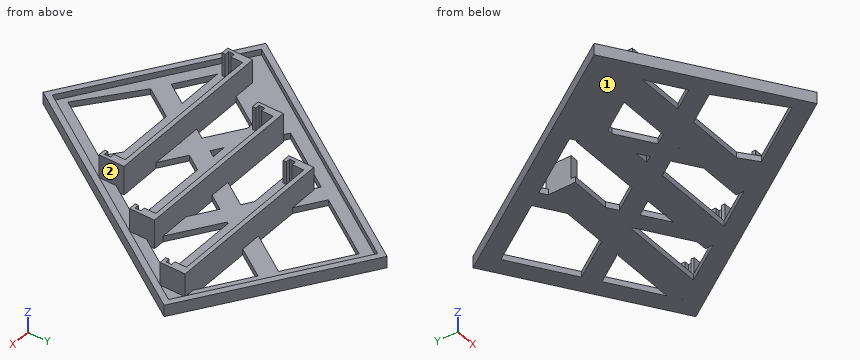
from build123d import *

# Parameters (mm, degrees)
PAD002_DEPTH = 4
PAD001_DEPTH = 10
SKETCH_W     = 59
SKETCH_H     = 10
PAD_DEPTH    = 2
PAD003_DEPTH = 2


with BuildPart() as pad002:
    # Sketch002 → Pad002 (new body)
    with BuildSketch(Plane.XY):
        Polygon((13.415017, 35.19739), (67.498286, -0.858122), (12.028266, -84.063152), (-42.055003, -48.007639), align=None)
        Polygon((13.969717, 32.423889), (-39.281502, -47.452939), (11.473566, -81.289651), (64.724785, -1.412822), align=None, mode=Mode.SUBTRACT)
    extrude(amount=PAD002_DEPTH)


with BuildPart() as pad001:
    # Sketch001 → Pad001 (new body)
    with BuildSketch(Plane.XY):
        Polygon((0, 0), (0, -8.6), (2.6, -8.6), (2.6, -7.5), (1.1, -7.5), (1.1, -5.5), (2.6, -5.5), (2.6, -1.5), (56.4, -1.5), (56.4, -5.5), (57.9, -5.5), (57.9, -7.5), (56.4, -7.5), (56.4, -8.6), (59, -8.6), (59, 0), align=None)
    extrude(amount=PAD001_DEPTH)


with BuildPart() as pad:
    # Sketch → Pad (new body)
    with BuildSketch(Plane.XY):
        with Locations((29.5, -5)):
            Rectangle(SKETCH_W, SKETCH_H)
    extrude(amount=PAD_DEPTH)


with BuildPart() as relay002:
    # Fusion001 base: copy of Pad
    add(pad.part)

    # Fusion001: union Pad001
    add(pad001.part)


with BuildPart() as relay002_1:
    # Fusion001 placement: moved
    add(relay002.part.moved(Location((-14, -21, 0))))


with BuildPart() as relay001:
    # Fusion base: copy of Pad
    add(pad.part)

    # Fusion: union Pad001
    add(pad001.part)


with BuildPart() as relay003:
    # Fusion002 base: copy of Pad
    add(pad.part)

    # Fusion002: union Pad001
    add(pad001.part)


with BuildPart() as relay003_1:
    # Fusion002 placement: moved
    add(relay003.part.moved(Location((-28, -42, 0))))


with BuildPart() as fusion003:
    # Sketch003 → Pad003 (new body)
    with BuildSketch(Plane.XY):
        Polygon((13.415017, 35.19739), (-42.055003, -48.007639), (12.028266, -84.063152), (67.498286, -0.858122), align=None)
        Polygon((15.079117, 26.876888), (34.632299, 13.841433), (20.579895, -7.237174), (1.026713, 5.79828), align=None, mode=Mode.SUBTRACT)
        Polygon((39.624601, 10.513232), (59.177783, -2.522223), (45.125378, -23.60083), (25.572196, -10.565375), align=None, mode=Mode.SUBTRACT)
        Polygon((-2.301489, 0.805979), (-16.353893, -20.272629), (3.199289, -33.308083), (17.251693, -12.229476), align=None, mode=Mode.SUBTRACT)
        Polygon((22.243995, -15.557677), (8.19159, -36.636284), (27.744772, -49.671739), (41.797177, -28.593132), align=None, mode=Mode.SUBTRACT)
        Polygon((0.059977, -38.426311), (-13.992428, -59.504919), (-26.473182, -51.184416), (-12.420777, -30.105808), align=None, mode=Mode.SUBTRACT)
        Polygon((5.054661, -41.750937), (-8.997744, -62.829544), (9.379179, -77.476683), (23.431584, -56.398076), align=None, mode=Mode.SUBTRACT)
    extrude(amount=PAD003_DEPTH)

    # Fusion003: union Pad002, Relay002, Relay001, Relay003
    add(pad002.part)
    add(relay002_1.part)
    add(relay001.part)
    add(relay003_1.part)


solid = fusion003.part
Here's how the part is built. I have some questions about the finished solid (model axes, mm). Face numbers are marked on the shaded views. Coordinates: 2 decimals unless noted, no trailing zeros. Loops run counter-clockwise (first coordinate to the right, second up) from the corner with the lowest first, then second, coordinate; pieces in that order, holes last. Notation, with made-up numbers: (-15, 82.25) -> (27, 82.25) arc R22 ccw to (27, 107.25) -> close; hole circle Ø11 at (82.25, -5.5). An arc over 180 degrees is marked (long way). Use one line per item in the form item = value. Start each with the question number.
(1) If we section it at B-B (y = -72.5): Please give me the cut outline in (x, z), then the cut area to 3 significant figures.
(2) We'd pull the mould along Y, two halves only. Please class the marked faces 1 and 2: pulls with the +Y half, pulls with the -Y half, needs draft (parallel to the pull), parting line crosses it, or undercut.
(3) Please list where these lines run through material, in increasing order: line 1 along Y through (x, z) = (29.5, 9.25); line 2 along Y through (x, z) = (16, 4.25); line 3 along Y through (x, z) = (-12, 4.5).
(4) If we section it at A-A (y = -35): Please give me the cut outline in (x, z).
(5) Will these pins go through, and if not, where does the flat tip stop? pin 1 (4 mm diameter, centred on y = -9.5, z = 2.5, fed in from +X); pin 2 (6 mm diameter, centred on y = -19, z = 8, fed in from +X); pin 3 (2 mm diameter, centred on x = 32.5, z = 1, fed in from -Y).
(6) If we section it at C-C (x = -6): Please give me the cut outline in (y, z).
(7) If we section it at D-D (z = 7.75): Give the number of separate pieces and of enclosed holes in the cut face, then the cut area to 3 significant figures.
Verdict:
q1.outline = (-5.32, 0) -> (3.14, 0) -> (3.14, 2) -> (-1.71, 2) -> (-1.71, 4) -> (-5.32, 4) -> close; (12.7, 0) -> (19.74, 0) -> (19.74, 4) -> (17.33, 4) -> (17.33, 2) -> (12.7, 2) -> close
q1.area = 43.0 mm²
q2.face_1 = needs draft
q2.face_2 = undercut
q3.line_1 = -50.6 to -49.5, -47.5 to -42, -22.5 to -21, -1.5 to 0
q3.line_2 = -43.5 to -42, -22.5 to -21, -1.5 to 0
q3.line_3 = -43.5 to -42, -29.6 to -28.5, -26.5 to -21
q4.outline = (-33.38, 0) -> (-15.68, 0) -> (-15.68, 2) -> (-30.98, 2) -> (-30.98, 4) -> (-33.38, 4) -> close; (-5.08, 0) -> (9.28, 0) -> (9.28, 2) -> (-5.08, 2) -> close; (37.53, 0) -> (44.74, 0) -> (44.74, 4) -> (42.33, 4) -> (42.33, 2) -> (37.53, 2) -> close
q5.pin_1 = 63.07
q5.pin_2 = 45
q5.pin_3 = -54.86
q6.outline = (-72.04, 0) -> (-65.22, 0) -> (-65.22, 2) -> (-69.64, 2) -> (-69.64, 4) -> (-72.04, 4) -> close; (-58.33, 0) -> (-42, 0) -> (-42, 10) -> (-43.5, 10) -> (-43.5, 2) -> (-58.33, 2) -> close; (-34.39, 0) -> (-21, 0) -> (-21, 10) -> (-22.5, 10) -> (-22.5, 2) -> (-34.39, 2) -> close; (-4.74, 0) -> (6.07, 0) -> (6.07, 4) -> (2.47, 4) -> (2.47, 2) -> (-4.74, 2) -> close
q7.separate_pieces = 3
q7.enclosed_holes = 0
q7.area = 358 mm²
